Source: CAD feature listing. Evaluate the final solid. Frame: model axes, mm. Face numbers are marked on the shaded views. A direction names the side the tool comes from. Give positions to 0.01 mm unless a question says otherwise; leave off trailing zeros. Loops run counter-clockwise (first coordinate to the right, second up) from the corner with the lowest first, then second, coordinate; pieces in that order, holes last.
```python
from build123d import *

# Parameters (mm, degrees)
BOSS_EXTRUDE1_DEPTH = 2
BOSS_EXTRUDE2_DEPTH = 10
SKETCH1_4_R         = 2.75
CUT_EXTRUDE1_DEPTH  = 2
FILLET1_R           = 2
SKETCH1_5_R         = 5.656929669
CUT_EXTRUDE5_DEPTH  = 0.25


with BuildPart() as part:
    # Sketch1 → Boss-Extrude1 (new body)
    with BuildSketch(Plane.XY):
        Polygon((-24.926279442, 5.5), (-24.926279442, -5.5), (-17.226279442, -9.945597073), (-17.226279442, -18.836791218), (-7.7, -24.336791218), (0, -19.891194146), (7.7, -24.336791218), (17.226279442, -18.836791218), (17.226279442, -7.836791218), (9.526279442, -3.391194146), (9.526279442, 5.5), (0, 11), (-7.7, 6.554402927), (-15.4, 11), align=None)
    extrude(amount=BOSS_EXTRUDE1_DEPTH)

    # Sketch1_3 → Boss-Extrude2 (add)
    with BuildSketch(Plane.XY):
        Polygon((0, 11), (9.526279442, 5.5), (9.526279442, -3.391194146), (17.226279442, -7.836791218), (17.226279442, -18.836791218), (7.7, -24.336791218), (0, -19.891194146), (-7.7, -24.336791218), (-17.226279442, -18.836791218), (-17.226279442, -9.945597073), (-24.926279442, -5.5), (-24.926279442, 5.5), (-15.4, 11), (-7.7, 6.554402927), align=None)
        Polygon((-15.4, 10.133974596), (-24.176279442, 5.066987298), (-24.176279442, -5.066987298), (-16.476279442, -9.512584371), (-16.476279442, -18.403778516), (-7.7, -23.470765814), (0, -19.025168742), (7.7, -23.470765814), (16.476279442, -18.403778516), (16.476279442, -8.26980392), (8.776279442, -3.824206847), (8.776279442, 5.066987298), (0, 10.133974596), (-7.7, 5.688377523), align=None, mode=Mode.SUBTRACT)
    extrude(amount=-BOSS_EXTRUDE2_DEPTH)

    # Sketch1_4 → Cut-Extrude1 (cut)
    with BuildSketch(Plane.XY):
        with Locations((-15.4, 0)):
            Circle(SKETCH1_4_R)
        Circle(SKETCH1_4_R)
        with Locations((-7.7, -13.336791218)):
            Circle(SKETCH1_4_R)
        with Locations((7.7, -13.336791218)):
            Circle(SKETCH1_4_R)
    extrude(amount=CUT_EXTRUDE1_DEPTH, mode=Mode.SUBTRACT)

    # Fillet1
    fillet1_edges = [part.edges().sort_by_distance(p)[0] for p in [
        (9.526279442, 1.054402927, 2),
        (13.376279442, -5.613992682, 2),
        (17.226279442, -13.336791218, 2),
        (12.463139721, -21.586791218, 2),
        (3.85, -22.113992682, 2),
        (-3.85, -22.113992682, 2),
        (-12.463139721, -21.586791218, 2),
        (-17.226279442, -14.391194146, 2),
        (-21.076279442, -7.722798536, 2),
        (-24.926279442, 0, 2),
        (-3.85, 8.777201464, 2),
        (-20.163139721, 8.25, 2),
        (-11.55, 8.777201464, 2),
        (4.763139721, 8.25, 2),
    ]]
    fillet(fillet1_edges, radius=FILLET1_R)

    # Sketch1_5 → Cut-Extrude5 (cut)
    with BuildSketch(Plane.XY):
        with Locations((-15.4, 0)):
            Circle(SKETCH1_5_R)
        Circle(SKETCH1_5_R)
        with Locations((7.7, -13.336791218)):
            Circle(SKETCH1_5_R)
        with Locations((-7.7, -13.336791218)):
            Circle(SKETCH1_5_R)
    extrude(amount=CUT_EXTRUDE5_DEPTH, mode=Mode.SUBTRACT)


solid = part.part
```
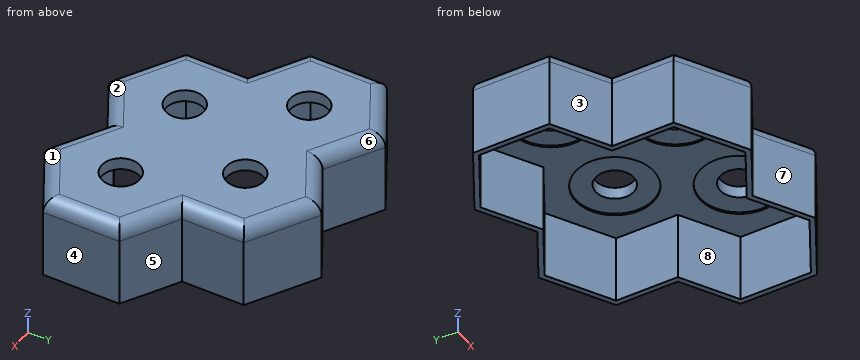
(1) Mould query, pull axis X, two halves, no side actions, for the marked faces 1, 2 and 3. Classes: pulls with the +X half, pulls with the -X half, needs draft (parallel to the pull), parting line crosses it, or undercut.
A:
face 1: pulls with the +X half
face 2: undercut
face 3: pulls with the -X half
(2) Section C-C, the plane y = -17. Return the cut outline in (x, z), then the cut area to 3 significant figures.
A:
outline: (-17.23, -10) - (-16.48, -10) - (-16.48, 0) - (-12.01, 0) - (-12.01, 0.25) - (-3.39, 0.25) - (-3.39, 0) - (3.39, 0) - (3.39, 0.25) - (12.01, 0.25) - (12.01, 0) - (16.48, 0) - (16.48, -10) - (17.23, -10) - (17.23, 0) arc R2 ccw to (15.23, 2) - (-15.23, 2) arc R2 ccw to (-17.23, 0) - close
area: 77.9 mm2
(3) Section B-B, the plane y = 0. Return the cut outline in (x, z).
A:
outline: (-24.93, -10) - (-24.18, -10) - (-24.18, 0) - (-21.06, 0) - (-21.06, 0.25) - (-18.15, 0.25) - (-18.15, 2) - (-22.93, 2) arc R2 ccw to (-24.93, 0) - close; (-12.65, 0.25) - (-9.74, 0.25) - (-9.74, 0) - (-5.66, 0) - (-5.66, 0.25) - (-2.75, 0.25) - (-2.75, 2) - (-12.65, 2) - close; (2.75, 0.25) - (5.66, 0.25) - (5.66, 0) - (8.78, 0) - (8.78, -10) - (9.53, -10) - (9.53, 0) arc R2 ccw to (7.53, 2) - (2.75, 2) - close
(4) Ray query, line 1 along X through (y, z) = (-1, -8.75); line 2 along X through (y, z) = (-17, -7.5); line 3 along X through (y, z) = (7.5, -2). Return the intervals inside material, ascending.
A:
line 1: x = -24.93 to -24.18, 8.78 to 9.53
line 2: x = -17.23 to -16.48, 16.48 to 17.23
line 3: x = -21.46 to -19.96, -10.84 to -9.34, -6.06 to -4.56, 4.56 to 6.06
(5) First-contact query: pin 1 (3 mm diameter, centred on y = 7.5, z = -7, fed in from -X); pin 2 (7 mm diameter, centred on x = -15.4, y = 0, fed in from -Z); pin 3 (2 mm diameter, centred on x = -6, y = 7, fed in from +Z). Flat tips, straight axial feed; report the tip coordinate or a pass-through.
A:
pin 1: stops at x = -24.06
pin 2: stops at z = 0.25
pin 3: stops at z = 1.93
(6) Section A-A, the plane z = -1.5. Return the cut outline in (x, y).
A:
outline: (-24.93, -5.5) - (-17.23, -9.95) - (-17.23, -18.84) - (-7.7, -24.34) - (0, -19.89) - (7.7, -24.34) - (17.23, -18.84) - (17.23, -7.84) - (9.53, -3.39) - (9.53, 5.5) - (0, 11) - (-7.7, 6.55) - (-15.4, 11) - (-24.93, 5.5) - close; hole (-24.18, -5.07) - (-16.48, -9.51) - (-16.48, -18.4) - (-7.7, -23.47) - (0, -19.03) - (7.7, -23.47) - (16.48, -18.4) - (16.48, -8.27) - (8.78, -3.82) - (8.78, 5.07) - (0, 10.13) - (-7.7, 5.69) - (-15.4, 10.13) - (-24.18, 5.07) - close
(7) Reachability of the marked faces 4, 5, 6, 7 and 8 from +Z, -Z, +X, -X, +Y, -Y: full face, straight path, thin tool, end or side. Return the list, or none.
A:
face 4: +Z, -Z, +X, +Y, -Y
face 5: +Z, -Z, +X, +Y
face 6: +Z, +Y
face 7: +Z, -Z, -Y
face 8: -Z
